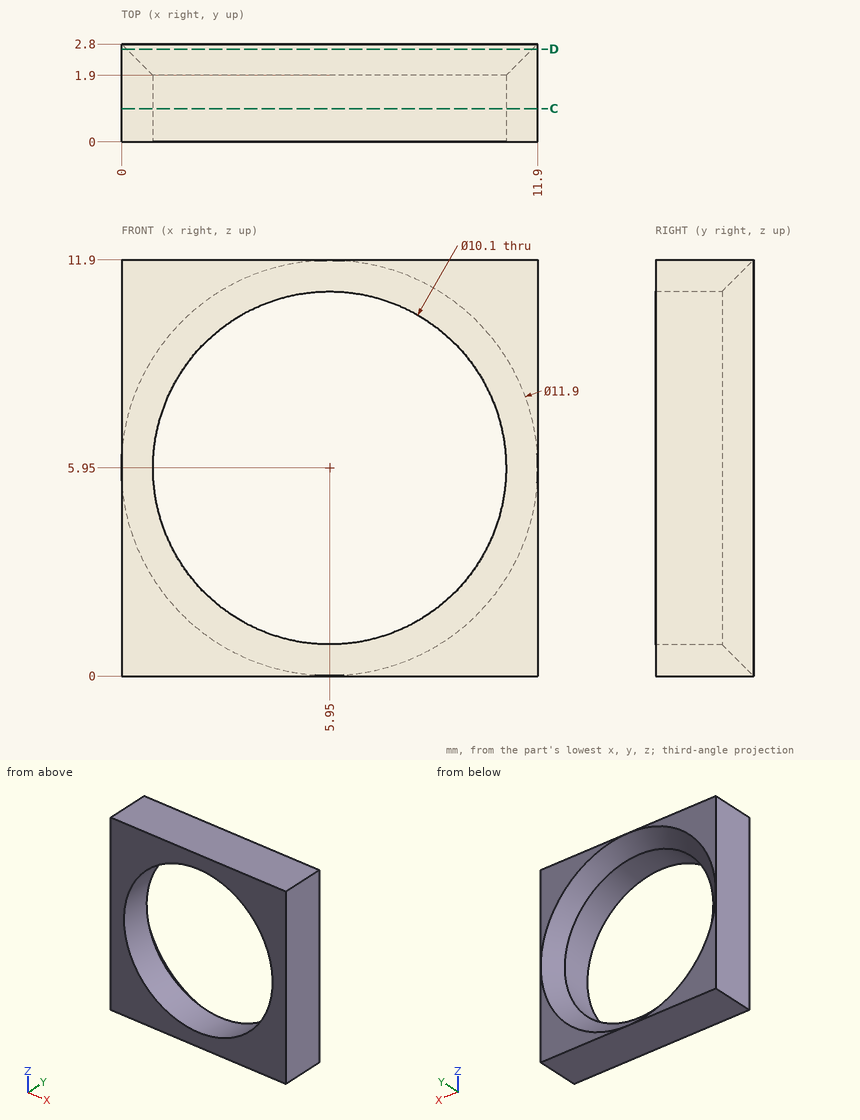
Answer from the drawing. Dimensions are ordinates in mm from the lowest x, y and z of the part. Round coordinates to 2 decimals unless told otherwise and drop trailing zeros. Write each loop counter-clockwise with the first axis right and the second up, starting at its lowest first coordinate (ties: lowest second). Pieces come first, ordered by that corner, then holes. Notation, with made-up numbers: (66, -37.5) - (106, -37.5) arc R16 cw to (106, -23.5) - close; hole circle Ø3 at (20.25, 24.5). An arc over 180 degrees is marked (long way). One line per item, written item: value.
Q1. Find section C-C (y = 0.95). Determine the outline of the cut face in (x, z), and give its area (3 significant figures).
The answers:
outline: (0, 0) - (11.9, 0) - (11.9, 11.9) - (0, 11.9) - close; hole circle Ø10.1 at (5.95, 5.95)
area: 61.5 mm2
Q2. Straight lines are drawn through the part: line 1 (X direction, y = 0.8, z = 5.95); line 2 (Z direction, x = 5.75, y = 2.35); line 3 (Z direction, x = 5.5, y = 1.85). For each, find the intervals that lie inside material, in ascending order. Write a range as from..to.
The answers:
line 1: x = 0..0.9, 11..11.9
line 2: z = 0..0.45, 11.45..11.9
line 3: z = 0..0.92, 10.98..11.9
Q3. Find section D-D (y = 2.65). Determine the outline of the cut face in (x, z).
The answers:
outline: (0, 0) - (11.9, 0) - (11.9, 11.9) - (0, 11.9) - close; hole circle Ø11.6 at (5.95, 5.95)
